Work out the finished part from the listing and answer in its coordinate system (mm). A direction names the side the tool comes from. Coordinates: 2 decimals unless noted, no trailing zeros. Loops run counter-clockwise (first coordinate to the right, second up) from the corner with the lowest first, then second, coordinate; pieces in that order, holes last. Notation, with made-up numbers: M 42,46 L 50,46 A16 ccw 50,57 Z; hole C -15.5,-3 d6. An arc over 180 degrees is marked long. Write each question's results on one line, items separated by ' | '.
```python
from build123d import *

# Parameters (mm, degrees)
ESBO_O1_R                  = 5
ESBO_O1_R_2                = 1.75
RESSALTO_EXTRUS_O1_DEPTH   = 10
ESBO_O2_W                  = 10
ESBO_O2_H                  = 2.5
RESSALTO_EXTRUS_O2_DEPTH   = 20
CORTE_EXTRUS_O1_DEPTH      = 15
CORTE_EXTRUS_O1_DEPTH_BACK = 14
ESBO_O3_R                  = 1.75
CORTE_EXTRUS_O3_DEPTH      = 12
CORTE_EXTRUS_O3_DEPTH_BACK = 14
ESBO_O5_W                  = 4
ESBO_O5_H                  = 14.425539271
FILETE1_R                  = 5
FILETE2_R                  = 5
CORTE_EXTRUS_O4_DEPTH      = 1.5
ESBO_O7_R                  = 3.25
CORTE_EXTRUS_O5_DEPTH      = 1.5


# Some blends are built 0.0001 mm under size
with BuildPart() as part:
    # Esboço1 → Ressalto-extrusão1 (new body)
    # profile 1 of 3: a face of its own
    with BuildSketch(Plane.XY):
        with BuildLine():
            ThreePointArc((0, -5), (-3.535533906, -3.535533906), (-5, 0))
            Line((-5, 0), (-5, -5))
            Line((-5, -5), (0, -5))
        make_face()
    # profile 2 of 3: a face of its own
    with BuildSketch(Plane.XY):
        Circle(ESBO_O1_R)
        Circle(ESBO_O1_R_2, mode=Mode.SUBTRACT)
    # profile 3 of 3: a face of its own
    with BuildSketch(Plane.XY):
        with BuildLine():
            Line((5, -5), (5, 0))
            ThreePointArc((5, 0), (3.535533906, -3.535533906), (0, -5))
            Line((0, -5), (5, -5))
        make_face()
    extrude(amount=RESSALTO_EXTRUS_O1_DEPTH)

    # Esboço2 → Ressalto-extrusão2 (add)
    with BuildSketch(Plane(origin=(5, 0, 5), x_dir=(0, 0, 1), z_dir=(-1, 0, 0))):
        with Locations((0, -6.25)):
            Rectangle(ESBO_O2_W, ESBO_O2_H)
    extrude(amount=RESSALTO_EXTRUS_O2_DEPTH)

    # Esboço3 → Corte-extrusão1 (cut, two sides: drawn at the far end of the back side and taken through both)
    with BuildSketch(Plane.XZ.offset(5).offset(-CORTE_EXTRUS_O1_DEPTH_BACK)):
        with Locations((-10, 5)):
            Circle(ESBO_O3_R)
    extrude(amount=CORTE_EXTRUS_O1_DEPTH + CORTE_EXTRUS_O1_DEPTH_BACK, mode=Mode.SUBTRACT)

    # Esboço5 → Corte-extrusão3 (cut, two sides: drawn at the far end of the back side and taken through both)
    with BuildSketch(Plane.ZY.offset(5).offset(-CORTE_EXTRUS_O3_DEPTH_BACK)):
        with Locations((5, 2.212769635)):
            Rectangle(ESBO_O5_W, ESBO_O5_H)
    extrude(amount=CORTE_EXTRUS_O3_DEPTH + CORTE_EXTRUS_O3_DEPTH_BACK, mode=Mode.SUBTRACT)

    # Filete1
    filete1_edges = [part.edges().sort_by_distance(p)[0] for p in [
        (-15, -6.25, 10),
        (-15, -6.25, 0),
    ]]
    fillet(filete1_edges, radius=FILETE1_R - 0.0001)  # a hair under: the kernel refuses the full size

    # Filete2
    # the kernel refuses this fillet: 5 mm, written as the material it takes off along each edge
    with BuildSketch(Plane(origin=(5, -7.5, 22.5), x_dir=(-1, 0, 0), z_dir=(0, 0, -1))) as filete2_piece_1:
        with BuildLine():
            CenterArc((FILETE2_R, FILETE2_R), FILETE2_R, 180, 90)
            Line((0, FILETE2_R), (0, 0))
            Line((0, 0), (FILETE2_R, 0))
        make_face()
    extrude(amount=35, mode=Mode.SUBTRACT)

    # Esboço6 → Corte-extrusão4 (cut)
    with BuildSketch(Plane(origin=(0, 0, 0), x_dir=(-1, 0, 0), z_dir=(0, 0, -1))):
        Polygon((0, 3.75277675), (-3.25, 1.876388375), (-3.25, -1.876388375), (0, -3.75277675), (3.25, -1.876388375), (3.25, 1.876388375), align=None)
    extrude(amount=-CORTE_EXTRUS_O4_DEPTH, mode=Mode.SUBTRACT)

    # Esboço7 → Corte-extrusão5 (cut)
    with BuildSketch(Plane.XY.offset(10)):
        Circle(ESBO_O7_R)
    extrude(amount=-CORTE_EXTRUS_O5_DEPTH, mode=Mode.SUBTRACT)


solid = part.part
```
1) For a pull along Z with two mould halves and no side action, classify faces 1 (the face through (1, -2, 1.5)), 2 (the face through (3.25, 0, 1)), 3 (the face through (-9.19, -6.23, 3.45)) as released by +Z, released by -Z, zero draft, split by the parting line, or undercut.
Check result:
face 1: released by -Z | face 2: zero draft | face 3: undercut
2) Find section D-D, the plane x = -9.5. Give the vertices of the cut face in (y, z).
Check result:
outline: M -7.5,0 L -5,0 L -5,3.32 L -7.5,3.32 Z; M -7.5,6.68 L -5,6.68 L -5,10 L -7.5,10 Z
3) Find section A-A, the plane x = -0.5. Give the vertices of the cut face in (y, z), and give its area (3 significant figures).
Check result:
outline: M -7.5,0 L -3.46,0 L -3.46,1.5 L -1.68,1.5 L -1.68,3 L -5,3 L -5,7 L -1.68,7 L -1.68,8.5 L -3.21,8.5 L -3.21,10 L -7.5,10 Z; M 1.68,1.5 L 3.46,1.5 L 3.46,0 L 4.97,0 L 4.97,3 L 1.68,3 Z; M 1.68,7 L 4.97,7 L 4.97,10 L 3.21,10 L 3.21,8.5 L 1.68,8.5 Z | area: 54.8 mm^2
4) Given pin 1 Ø1.2 at (y, z) = (0, 0.5) entering from -X; pin 2 Ø3 at (x, z) = (-2, 3.5) entering from +Y; pin 3 Ø4 at (x, y) = (0, 0) entering from -Z, each flat-ended and moving along its own axis, determine where each tip first touches the part or whether it passes through.
Check result:
pin 1: x = -5 | pin 2: y = 4.97 | pin 3: z = 1.5
5) Which of the six approach directions +Z, -Z, +X, -X, +Y, -Y give full straight-line access (tool end or side, diameter ignored) to faces 4 (the face through (0, -2, 3)), 5 (the face through (1.6, 2.83, 0.74)), 6 (the face through (1.4, -1.4, 8.5))?
Check result:
face 4: +X, -X, +Y | face 5: -Z | face 6: +Z
6) Straight lines are drawn through the part: probe 1 along Y at (x, z) = (0, 8.9); probe 2 along Z at (x, y) = (-10, -5.75); probe 3 along Y at (x, z) = (0, 7.55). For each, find the intervals that lie inside material, in ascending order. Write a range as [from, to].
Check result:
probe 1: [-7.5, -3.25], [3.25, 5] | probe 2: [0, 3.25], [6.75, 10] | probe 3: [-7.5, -1.75], [1.75, 5]
7) Find section C-C, the plane z = 3.5. Give the vertices of the cut face in (x, y), and give its area (3 significant figures).
Check result:
outline: M -14.77,-7.5 L -10.9,-7.5 L -10.9,-5 L -14.77,-5 Z; M -9.1,-7.5 L 0,-7.5 A5 ccw 4.33,-5 L -9.1,-5 Z | area: 40.1 mm^2
8) Find section B-B, the plane y = 3. Give the vertices of the cut face in (x, z), and give its area (3 significant figures).
Check result:
outline: M -4,0 L -1.3,0 L -1.3,1.5 L 1.3,1.5 L 1.3,0 L 4,0 L 4,3 L -4,3 Z; M -4,7 L 4,7 L 4,10 L 1.25,10 L 1.25,8.5 L -1.25,8.5 L -1.25,10 L -4,10 Z | area: 40.3 mm^2
